Design review of the part built by this model. Coordinates are the model's own, in mm. Face numbers are marked on the shaded views. A direction names the side the tool comes from. Give positions to 0.01 mm unless a question says otherwise; leave off trailing zeros. Order: outer loops, then holes, each group sorted by start corner. A loop starts at its lowest first (then second) coordinate and runs counter-clockwise, first axis right, second up.
```python
from build123d import *

# Parameters (mm, degrees)
SKETCH1_W                = 25.4
SKETCH1_H                = 6.35
FILLET1_R                = 10.16
BOSS_EXTRUDE1_DEPTH      = 38.1
BOSS_EXTRUDE1_DEPTH_BACK = 20.32
SKETCH3_W                = 25.4
SKETCH3_H                = 12.7
SKETCH4_W                = 25.4
SKETCH4_H                = 12.7
BOSS_EXTRUDE2_DEPTH      = 76.2
SKETCH5_R                = 3.175
CUT_EXTRUDE1_DEPTH       = 159.762008669


with BuildPart() as part:
    # Sketch1 → Revolve1 (revolve)
    with BuildSketch(Plane.XY, mode=Mode.PRIVATE) as revolve1_sk:
        Polygon((0, 48.048104246), (0, 22.664551268), (25.4, 22.664551268), (17.22966458, 48.048104246), align=None)
        Polygon((0, 22.664551268), (0, 20.09296726), (25.4, 20.09296726), (38.1, 20.09296726), (38.1, 22.664551268), (25.4, 22.664551268), align=None)
        with Locations((12.7, 16.91796726)):
            Rectangle(SKETCH1_W, SKETCH1_H)
    revolve(revolve1_sk.sketch.rotate(Axis((0, 27.702147105, 0), (0, -1, 0)), 90), axis=Axis((0, 27.702147105, 0), (0, -1, 0)))

    # Sketch2 → Revolve2 (revolve)
    with BuildSketch(Plane(origin=(0, 0, 0), x_dir=(0, 0, -1), z_dir=(1, 0, 0))):
        with BuildLine():
            Line((0, 48.048104246), (17.22966458, 48.048104246))
            add(Edge.make_bspline(
                [(17.22966458, 48.048104246), (8.61483229, 61.740341407), (0, 61.740341407)],
                knots=[0, 0, 0, 0.5, 0.5, 0.5], degree=2))
            Line((0, 61.740341407), (0, 48.048104246))
        make_face()
    revolve(axis=Axis((0, 0, 0), (0, 1, 0)))

    # Fillet1
    fillet1_edges = [part.edges().sort_by_distance(p)[0] for p in [
        (-17.22966458, 48.048104246, 0),
    ]]
    fillet(fillet1_edges, radius=FILLET1_R)

    # Sketch3 → Boss-Extrude1 (add, two sides: drawn at the far end of the back side and taken through both)
    with BuildSketch(Plane(origin=(22.86, 0, 0), x_dir=(0, 0, -1), z_dir=(1, 0, 0)).offset(-BOSS_EXTRUDE1_DEPTH_BACK)):
        with Locations((0, 46.783028789)):
            Rectangle(SKETCH3_W, SKETCH3_H)
    extrude(amount=BOSS_EXTRUDE1_DEPTH + BOSS_EXTRUDE1_DEPTH_BACK)

    # Sketch4 → Boss-Extrude2 (add)
    with BuildSketch(Plane(origin=(60.96, 0, 0), x_dir=(0, 0, -1), z_dir=(1, 0, 0))):
        with Locations((0, 46.783028789)):
            Rectangle(SKETCH4_W, SKETCH4_H)
    extrude(amount=BOSS_EXTRUDE2_DEPTH)

    # Sketch5 → Cut-Extrude1 (cut, through all)
    with BuildSketch(Plane(origin=(0, 0, -12.7), x_dir=(-1, 0, 0), z_dir=(0, 0, -1))):
        with Locations((-130.81, 46.783028789)):
            Circle(SKETCH5_R)
        with Locations((-118.11, 46.783028789)):
            Circle(SKETCH5_R)
        with Locations((-105.41, 46.783028789)):
            Circle(SKETCH5_R)
    extrude(amount=-CUT_EXTRUDE1_DEPTH, mode=Mode.SUBTRACT)


solid = part.part
```
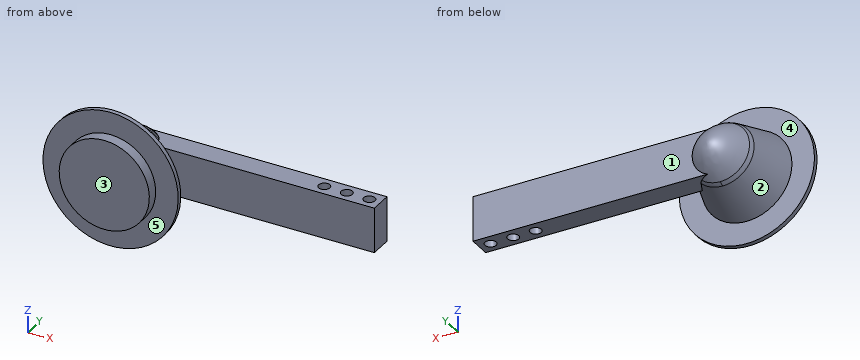
1. Machinability: for the marked faces 4 and 5, which of the approach directions +Z, -Z, +X, -X, +Y, -Y give a long, thin tool a straight path to every point of the face, cutting with its end or side? Answer none if there is none.
Recorded:
face 4: none
face 5: -Y
2. Take a section at D-D (z = -31). State the section outline as (x, y) points.
Recorded:
outline: (-22.15, 20.09) - (22.15, 20.09) - (22.15, 22.66) - (-22.15, 22.66) - close
3. Take a section at C-C (y = 33). State the section outline as (x, z) points.
Recorded:
outline: circle Ø44.15 at (0, 0)
4. For pin 1 (8.5 mm diameter, centred on x = 118.11, y = 46.78, fed in from +Z); pin 2 (12.5 mm diameter, centred on x = 84.5, z = -3, fed in from -Y); pin 3 (3 mm diameter, centred on x = 56.5, z = 1, fed in from +Y), all flat-tipped, find the tip position at first contact; note any pin that passes through.
Recorded:
pin 1: stops at z = 12.7
pin 2: stops at y = 40.43
pin 3: stops at y = 53.13
5. Take a section at B-B (z = -4.5). State how many separate pieces and enclosed holes the cut face has, then the cut area to 3 significant figures.
Recorded:
separate pieces: 1
enclosed holes: 3
area: 3,290 mm2
6. For line 1 along X through (y, z) = (47.5, 11.5); line 2 along Z through (x, y) = (14, 46.5); line 3 along Y through (x, z) = (105, 0), list the stretches that pass through material, from the lowest coordinate up.
Recorded:
line 1: x = -13.03 to 102.32, 108.5 to 115.02, 121.2 to 127.72, 133.9 to 137.16
line 2: z = -12.7 to 12.7
line 3: y = 40.43 to 43.63, 49.93 to 53.13
7. Draft analysis for pull direction Y (two halves, no side actions). For the marked faces 1, 2 and 3, state which applies: pulls with the +Y half, pulls with the -Y half, needs draft (parallel to the pull), parting line crosses it, or undercut.
Recorded:
face 1: pulls with the +Y half
face 2: undercut
face 3: pulls with the -Y half
8. Take a section at A-A (x = 130.81). State the section outline as (y, z) points.
Recorded:
outline: (40.43, -12.7) - (43.61, -12.7) - (43.61, 12.7) - (40.43, 12.7) - close; (49.96, -12.7) - (53.13, -12.7) - (53.13, 12.7) - (49.96, 12.7) - close
